```python
from build123d import *

# Parameters (mm, degrees)
F1_W     = 130
F1_H     = 90
F3_DEPTH = 10
F2_R     = 2.5
F4_DEPTH = 10.001
F0_R     = 3
F0_R_2   = 2
F5_DEPTH = 10.001
F6_R     = 3
F7_DEPTH = 10.001
F9_DEPTH = 10.001


with BuildPart() as f3:
    # F1 (on Front) → F3 (new body)
    with BuildSketch(Plane.XZ):
        with Locations((0, -13)):
            Rectangle(F1_W, F1_H)
    extrude(amount=F3_DEPTH)

    # F2 (on Front) → F4 (cut, through all)
    with BuildSketch(Plane.XZ):
        with Locations((23, -6)):
            Circle(F2_R)
        with Locations((23, 12)):
            Circle(F2_R)
        with Locations((-23, -6)):
            Circle(F2_R)
        with Locations((-23, 12)):
            Circle(F2_R)
    extrude(amount=F4_DEPTH, mode=Mode.SUBTRACT)

    # F0 (on Front) → F5 (cut, through all)
    with BuildSketch(Plane.XZ):
        with Locations((-36, 0)):
            Circle(F0_R)
        with Locations((36, 0)):
            Circle(F0_R)
        with Locations((-55, -1)):
            Circle(F0_R_2)
        with Locations((55, -1)):
            Circle(F0_R_2)
        with BuildLine():
            ThreePointArc((18, 14), (16.535534, 17.535534), (13, 19))
            Line((13, 19), (-13, 19))
            ThreePointArc((-13, 19), (-16.535534, 17.535534), (-18, 14))
            Line((-18, 14), (-18, -26))
            ThreePointArc((-18, -26), (-16.535534, -29.535534), (-13, -31))
            Line((-13, -31), (13, -31))
            ThreePointArc((13, -31), (16.535534, -29.535534), (18, -26))
            Line((18, -26), (18, 14))
        make_face()
    extrude(amount=F5_DEPTH, mode=Mode.SUBTRACT)

    # F6 (on Front) → F7 (cut, through all)
    with BuildSketch(Plane.XZ):
        with Locations((34.8, -47.8)):
            Circle(F6_R)
        with Locations((34.8, 21.8)):
            Circle(F6_R)
        with Locations((-34.8, -47.8)):
            Circle(F6_R)
        with Locations((-34.8, 21.8)):
            Circle(F6_R)
    extrude(amount=F7_DEPTH, mode=Mode.SUBTRACT)

    # F8 (on Front) → F9 (cut, through all)
    with BuildSketch(Plane.XZ):
        with BuildLine():
            Line((-65, -18), (-65, -58))
            Line((-65, -58), (-45, -58))
            Line((-45, -58), (-45, -23))
            ThreePointArc((-45, -23), (-46.464466, -19.464466), (-50, -18))
            Line((-50, -18), (-65, -18))
        make_face()
        with BuildLine():
            Line((45, -58), (65, -58))
            Line((65, -58), (65, -18))
            Line((65, -18), (50, -18))
            ThreePointArc((50, -18), (46.464466, -19.464466), (45, -23))
            Line((45, -23), (45, -58))
        make_face()
    extrude(amount=F9_DEPTH, mode=Mode.SUBTRACT)


solid = f3.part
```
Build history of the part. All positions in model axes, mm. A direction names the side the tool comes from. Round coordinates to 2 decimals unless told otherwise and drop trailing zeros. Order: outer loops, then holes, each group sorted by start corner. A loop starts at its lowest first (then second) coordinate and runs counter-clockwise, first axis right, second up. Notation, with made-up numbers: (31.5, 19.25) - (86.5, 19.25) arc R25 ccw to (86.5, 58.25) - close; hole circle Ø2 at (-20.5, 1.25). An arc over 180 degrees is marked (long way). Use a Markdown table: item, result.
1) Saw through at C-C on x = -0.5. Write the cut outline in (y, z), and give its area (3 significant figures).
Recorded:
| item | result |
|---|---|
| outline | (-10, -58) - (0, -58) - (0, -31) - (-10, -31) - close; (-10, 19) - (0, 19) - (0, 32) - (-10, 32) - close |
| area | 400 mm² |
2) Tool access for faces 4 (the face through (0, -5, -31)), 5 (the face through (-45, -5, -41)), 6 (the face through (-65, -5, 7)), 7 (the face through (65, -5, 7)), 8 (the face through (58, -5, -18)): list every direction of +Z, -Z, +X, -X, +Y, -Y with a clear straight run to the whole face (end or side of a thin tool).
Recorded:
| item | result |
|---|---|
| face 4 | +Y, -Y |
| face 5 | -Z, -X, +Y, -Y |
| face 6 | +Z, -Z, -X, +Y, -Y |
| face 7 | +Z, -Z, +X, +Y, -Y |
| face 8 | -Z, +X, +Y, -Y |
3) Pull direction Z, two halves, no side cores. Call faces 1 (the face through (-57, -5, -18)), 2 (the face through (-1, 0, -32)), 3 (the face through (-25.5, -4.9, -5.9)): pulls with the +Z half, pulls with the -Z half, needs draft (parallel to the pull), parting line crosses it, or undercut.
Recorded:
| item | result |
|---|---|
| face 1 | pulls with the -Z half |
| face 2 | needs draft |
| face 3 | undercut |
4) Saw through at B-B on x = -23. Write the cut outline in (y, z).
Recorded:
| item | result |
|---|---|
| outline | (-10, -58) - (0, -58) - (0, -8.5) - (-10, -8.5) - close; (-10, -3.5) - (0, -3.5) - (0, 9.5) - (-10, 9.5) - close; (-10, 14.5) - (0, 14.5) - (0, 32) - (-10, 32) - close |
5) Wall check: L1, parallel to X at y = -4.25, z = 21.8; L2, parallel to X at y = -2.75, z = 12; L3, parallel to X at y = -6, z = -47.8. Give the ranges that are in metal, low to high.
Recorded:
| item | result |
|---|---|
| L1 | x = -65 to -37.8, -31.8 to 31.8, 37.8 to 65 |
| L2 | x = -65 to -25.5, -20.5 to -18, 18 to 20.5, 25.5 to 65 |
| L3 | x = -45 to -37.8, -31.8 to 31.8, 37.8 to 45 |
6) Saw through at A-A on z = 12. Write the cut outline in (x, y), and give its area (3 significant figures).
Recorded:
| item | result |
|---|---|
| outline | (-65, -10) - (-25.5, -10) - (-25.5, 0) - (-65, 0) - close; (-20.5, -10) - (-18, -10) - (-18, 0) - (-20.5, 0) - close; (18, -10) - (20.5, -10) - (20.5, 0) - (18, 0) - close; (25.5, -10) - (65, -10) - (65, 0) - (25.5, 0) - close |
| area | 840 mm² |
7) Flat gauge pins, fed straight in: pin 1 Ø10 at (x, z) = (37.5, -10.5) entering from +Y; pin 2 Ø5 at (x, y) = (-61, -2.5) entering from -Z; pin 3 Ø6 at (y, z) = (-8, -40) entering from -X. Where does each tip first touch, or does it go through?
Recorded:
| item | result |
|---|---|
| pin 1 | stops at y = 0 |
| pin 2 | stops at z = -18 |
| pin 3 | stops at x = -45 |
8) Saw through at D-D on z = -11.5. Write the cut outline in (x, y).
Recorded:
| item | result |
|---|---|
| outline | (-65, -10) - (-18, -10) - (-18, 0) - (-65, 0) - close; (18, -10) - (65, -10) - (65, 0) - (18, 0) - close |
